Input: part model. Units: mm. Frame: model coordinates. Face numbers are marked on the shaded views. Give positions to 0.01 mm unless a question says otherwise; leave off trailing zeros. Loops run counter-clockwise (first coordinate to the right, second up) from the corner with the lowest first, then second, coordinate; pieces in that order, holes last. Notation, with made-up numbers: (-26.5, 84.25) - (22.5, 84.25) arc R15 ccw to (22.5, 101.25) - close; hole circle Ø3 at (78, -16.75). An arc over 180 degrees is marked (long way). One line per item, written item: value.
from build123d import *

# Parameters (mm, degrees)
BOSS_EXTRUDE1_DEPTH = 140


with BuildPart() as part:
    # Sketch1 → Boss-Extrude1 (new body)
    with BuildSketch(Plane(origin=(0, 0, 0), x_dir=(1, 0, 0), z_dir=(0, 1, 0))):
        Polygon((-12.071067812, -5), (-12.071067812, 5), (-5, 12.071067812), (5, 12.071067812), (12.071067812, 5), (12.071067812, -5), (5, -12.071067812), (-5, -12.071067812), align=None)
    extrude(amount=BOSS_EXTRUDE1_DEPTH)

    # Sketch3 → Cut-Revolve2 (revolve, cut)
    with BuildSketch(Plane.XY):
        Polygon((1.5, 140), (14.42266182, 117.617293159), (14.42266182, 140), align=None)
    revolve(axis=Axis((0, 140, 0), (0, -1, 0)), mode=Mode.SUBTRACT)

    # Sketch4 → Revolve1 (revolve)
    with BuildSketch(Plane.XY):
        with BuildLine():
            Line((0, 145.598076211), (0, 140))
            Line((0, 140), (1.5, 140))
            ThreePointArc((1.5, 140), (2.897777479, 143.374533347), (0, 145.598076211))
        make_face()
    revolve(axis=Axis((0, 145.598076211, 0), (0, -1, 0)))

    # Sketch5 → Cut-Revolve3 (revolve, cut)
    with BuildSketch(Plane.XY):
        Polygon((0, 0), (5, 0), (5, 110), (0, 118.660254038), align=None)
    revolve(axis=Axis((0, 118.660254038, 0), (0, -1, 0)), mode=Mode.SUBTRACT)


solid = part.part
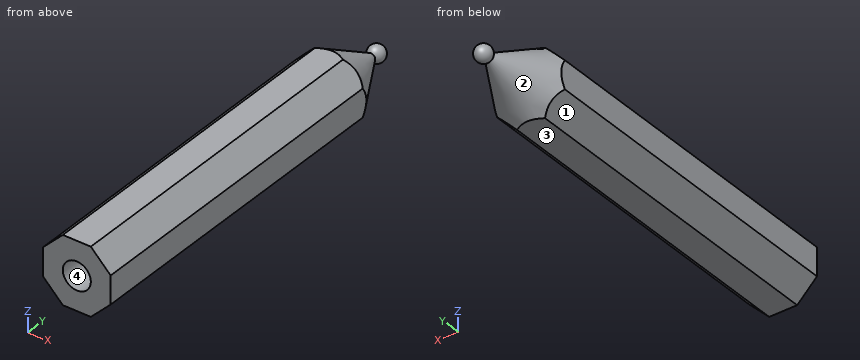
Item 1: Section A-A, the plane y = 98.5. Output: boundary loops of the cut face in (x, z).
Verdict:
outline: (-12.07, -5) - (-5, -12.07) - (5, -12.07) - (12.07, -5) - (12.07, 5) - (5, 12.07) - (-5, 12.07) - (-12.07, 5) - close; hole circle Ø10 at (0, 0)
Item 2: Draft query along X for the marked faces 1, 2, 3 and 4. Return one class per face: pulls with the +X half, pulls with the -X half, needs draft (parallel to the pull), parting line crosses it, or undercut.
Verdict:
face 1: pulls with the -X half
face 2: parting line crosses it
face 3: needs draft
face 4: undercut
Item 3: Material intervals for L1, parallel to Z at x = 0, y = 28.5; L2, parallel to X at y = 96, z = -4; L3, parallel to Z at x = 2.25, y = 65.5, sorted ascending.
Verdict:
L1: z = -12.07 to -5, 5 to 12.07
L2: x = -12.07 to -3, 3 to 12.07
L3: z = -12.07 to -4.47, 4.47 to 12.07
Item 4: Pin query (flat end, axial travel): P1, Ø8, axis at x = 9.5, y = 57.5, coming from the -Z side; P2, Ø8, axis at x = 9, z = -6.5, coming from the +Y side; P3, Ø5, axis at y = 23, z = -9, coming from the -X side. Return the tip coordinate at first contact, or that it passes through.
Verdict:
P1: stops at z = -11.57
P2: stops at y = 130.3
P3: stops at x = -10.57
